from build123d import *

# Parameters (mm, degrees)
SKETCH_2_R          = 1.100000024
EXTRUDE_1_DEPTH     = 4
SKETCH_4_R          = 1
CUT_EXTRUDE_1_DEPTH = 5
CUT_EXTRUDE_2_DEPTH = 5


with BuildPart() as part:
    # 草图2 → 凸台-拉伸1 (new body)
    with BuildSketch(Plane.XY):
        with BuildLine():
            Line((5.998458769, 1.854285714), (-7.998458769, 1.854285714))
            Line((-7.998458769, 1.854285714), (-7.998458769, -2.145714286))
            Line((-7.998458769, -2.145714286), (5.998458769, -2.145714286))
            ThreePointArc((5.998458769, -2.145714286), (7.998458769, -0.145714286), (5.998458769, 1.854285714))
        make_face()
        with Locations((5.998458956, -0.145714128)):
            Circle(SKETCH_2_R, mode=Mode.SUBTRACT)
    extrude(amount=EXTRUDE_1_DEPTH)

    # 草图4 → 切除-拉伸1 (cut)
    with BuildSketch(Plane.ZY.offset(7.998458769)):
        with Locations((2, -0.145714286)):
            Circle(SKETCH_4_R)
    extrude(amount=-CUT_EXTRUDE_1_DEPTH, mode=Mode.SUBTRACT)

    # 草图6 → 切除-拉伸2 (cut)
    with BuildSketch(Plane(origin=(0, 1.854285714, 0), x_dir=(1, 0, 0), z_dir=(0, 1, 0))):
        with BuildLine():
            Line((0.430237449, -2), (8.42228294, -2))
            Line((8.42228294, -2), (8.42228294, -4.483544919))
            Line((8.42228294, -4.483544919), (-3.767400724, -4))
            add(Edge.make_bspline(
                [(-3.767400724, -4), (-2.756163947, -3.891783592), (-1.123117091, -3.429006158), (-0.148462867, -2.077202756), (0.430237449, -2)],
                knots=[0, 0, 0, 0, 0.656759568, 1, 1, 1, 1], degree=3))
        make_face()
    extrude(amount=-CUT_EXTRUDE_2_DEPTH, mode=Mode.SUBTRACT)


solid = part.part
Source: CAD feature listing. Evaluate the final solid. Frame: model axes, mm. A direction names the side the tool comes from. Coordinates: 2 decimals unless noted, no trailing zeros. Order: outer loops, then holes, each group sorted by start corner. A loop starts at its lowest first (then second) coordinate and runs counter-clockwise, first axis right, second up.
Item 1: Cut plane B-B (x = 5.5). Return loops of the section in (y, z), plus the area to 3 significant figures.
Output values:
outline: (-2.15, 0) - (-1.13, 0) - (-1.13, 2) - (-2.15, 2) - close; (0.83, 0) - (1.85, 0) - (1.85, 2) - (0.83, 2) - close
area: 4.08 mm2
Item 2: Material intervals for line 1 (Y direction, x = -5.3, z = 2); line 2 (Z direction, x = -6.5, y = -0.15); line 3 (Z direction, x = -5, y = -0.55), sorted ascending.
Output values:
line 1: y = -2.15 to -1.15, 0.85 to 1.85
line 2: z = 0 to 1, 3 to 4
line 3: z = 0 to 1.09, 2.91 to 4
Item 3: Cut plane C-C (x = 1.25). Return loops of the section in (y, z), plus the area to 3 significant figures.
Output values:
outline: (-2.15, 0) - (1.85, 0) - (1.85, 2) - (-2.15, 2) - close
area: 8.00 mm2
Item 4: Pull-direction query (Y, two-part tool) for faces 3 (the face through (5.13, -0.82, 0.99)), 4 (the face through (3, 0, 2)), 5 (the face through (-3, -2.146, 2)); classes: pulls with the +Y half, pulls with the -Y half, needs draft (parallel to the pull), parting line crosses it, or undercut.
Output values:
face 3: undercut
face 4: needs draft
face 5: pulls with the -Y half
Item 5: Cut plane A-A (z = 0.5). Return loops of the section in (x, y).
Output values:
outline: (-8, -2.15) - (6, -2.15) arc R2 ccw to (6, 1.85) - (-8, 1.85) - close; hole circle Ø2.2 at (6, -0.15)
Item 6: Cut plane D-D (x = -6.25). Return loops of the section in (y, z).
Output values:
outline: (-2.15, 0) - (1.85, 0) - (1.85, 4) - (-2.15, 4) - close; hole circle Ø2 at (-0.15, 2)
Item 7: Set-up query: faces 1 (the face through (-2.998, 0, 2)), 2 (the face through (0, 0, 0)). Return all of +Z, -Z, +X, -X, +Y, -Y with unobstructed straight access to the full face (end or side cutting, diameter ignored); none if empty.
Output values:
face 1: -X
face 2: -Z, +X, -X, +Y, -Y
Item 8: First-contact query: P1, Ø2, axis at x = 4.5, y = 0, coming from the +Z side. Flat tip, straight axial feed; report the tip coordinate or a pass-through.
Output values:
P1: stops at z = 2
